CAD build for the part. Positions are in the model's coordinates, mm. Give positions to 0.01 mm unless a question says otherwise; leave off trailing zeros. Order: outer loops, then holes, each group sorted by start corner. A loop starts at its lowest first (then second) coordinate and runs counter-clockwise, first axis right, second up. Notation, with made-up numbers: (17, 1) -> (56, 1) arc R24 cw to (56, 33) -> close; hole circle Ø10 at (76, 67.25). An arc over 180 degrees is marked (long way). Answer as CSV lines item,"result".
Autodesk Inventor part; units mm, degrees
ref_plane "YZ Plane" through (0, 0, 0) normal (1, 0, 0) x (0, 1, 0)
ref_plane "XZ Plane" through (0, 0, 0) normal (0, 1, 0) x (-1, 0, 0)
ref_plane "XY Plane" through (0, 0, 0) normal (0, 0, 1) x (1, 0, 0)
sketch "Sketch1" plane through (0, 0, 0) normal (0, 0, 1) x (1, 0, 0)
  arc A0 (3.3974, 9.4052) -> (9.3315, -3.5948) centre (0, 0) ccw
  line L0 (3.3974, 9.4052) -> (29.434, 0)
  line L1 (9.3315, -3.5948) -> (29.434, 0)
  dimension "d0" = 20
  dimension "d33" = 30
  dimension "d34" = 13
extrude "Extrusion1" add sketch "Sketch1" along normal blind 7
sketch "Sketch2" plane through (0, 0, 7) normal (0, 0, 1) x (1, 0, 0)
  arc A0 (3.3974, 9.4052) -> (9.3315, -3.5948) centre (0, 0) ccw
  point P0 (0, -2)
  dimension "d12" = 2
hole "Hole1" at (0, -2, 7) direction (0, 0, -1) diameter 10.5 depth 8 tip angle 118
fillet "Fillet1" radius 2 1 edges at (29.434, 0, 3.5)
fillet "Fillet2" radius 6 1 edges at (9.3315, -3.5948, 3.5)
fillet "Fillet3" radius 1 8 edges at (-9.5121, -3.0855, 7) (17.1322, -2.1999, 7) (23.7272, 0.4854, 7) (12.9056, 5.9705, 7) (23.7272, 0.4854, 0) (12.9056, 5.9705, 0) (-9.5121, -3.0855, 0) (17.1322, -2.1999, 0)
properties part number "ExtruderQuickReleaseTensionCam" material "ABS Plastic"
1) Band-saw the part on A-A, the plane z = 1.75. Write the cut outline in (x, y).
Data:
outline,"(3.4, 9.41) arc R10 ccw (long way) to (8.27, -5.62) arc R6 cw to (12.18, -3.09) -> (22.09, -1.31) arc R2 ccw to (22.41, 2.54) -> close; hole circle Ø10.5 at (0, -2)"
2) Wall check: line 1 along Y through (x, z) = (0, 2.5); line 2 along Y through (x, z) = (4.5, 6.75); line 3 along Y through (x, z) = (11.5, 6.5). Give the ranges that are in metal, low to high. Write a range as [from, to].
Data:
line 1,"y = [-10, -7.25], [3.25, 10]"
line 2,"y = [-8.55, -4.7], [0.7, 8.65]"
line 3,"y = [-3.11, 6.34]"
3) Pin check, flat tips, straight feed: P1, Ø1, axis at x = 5, z = 2.5, coming from the +Y side; P2, Ø5, axis at x = -0.5, y = 4, coming from the -Z side; P3, Ø2, axis at y = -3, z = 5.5, coming from the -X side; P4, Ø1, axis at x = 19.5, z = 3.5, coming from the -Y side. Stop position of each tip, or through.
Data:
P1,"stops at y = 9.01"
P2,"stops at z = 0"
P3,"stops at x = -9.8"
P4,"stops at y = -1.87"
4) Pull direction X, two halves, no side cores. Call faces 1 (the cylindrical face through (17.01, -1.92, 0.29)), 2 (the flat face through (7, 0, 7)), 3 (the cylindrical face through (-1.6, -7, 3.5)): pulls with the +X half, pulls with the -X half, needs draft (parallel to the pull), parting line crosses it, or undercut.
Data:
face 1,"pulls with the +X half"
face 2,"needs draft"
face 3,"undercut"
